Model file for the job. Use its own axes, mm. A direction names the side the tool comes from. Coordinates: 2 decimals unless noted, no trailing zeros. Loops run counter-clockwise (first coordinate to the right, second up) from the corner with the lowest first, then second, coordinate; pieces in that order, holes last. Notation, with made-up numbers: (-30.5, 76) -> (12.5, 76) arc R25 ccw to (12.5, 113) -> close; hole circle Ø10 at (48, 87). An arc over 180 degrees is marked (long way). Use one line per item in the form item = value.
```python
from build123d import *

# Parameters (mm, degrees)
ESBO_O1_W                = 44
ESBO_O1_H                = 65
RESSALTO_EXTRUS_O1_DEPTH = 19
ESBO_O2_W                = 40
ESBO_O2_H                = 15
CORTE_EXTRUS_O1_DEPTH    = 20
ESBO_O3_W                = 40
ESBO_O3_H                = 1.8
CORTE_EXTRUS_O2_DEPTH    = 43
ESBO_O4_W                = 33
ESBO_O4_H                = 7.6
CORTE_EXTRUS_O3_DEPTH    = 43
ESBO_O5_W                = 3.5
ESBO_O5_H                = 7.6
RESSALTO_EXTRUS_O2_DEPTH = 20
ESBO_O6_W                = 33
ESBO_O6_H                = 5.6
CORTE_EXTRUS_O4_DEPTH    = 43
ESBO_O7_W                = 3.5
ESBO_O7_H                = 2
ESBO_O7_W_2              = 40
CORTE_EXTRUS_O5_DEPTH    = 63
ESBO_O8_R                = 2.05
CORTE_EXTRUS_O6_DEPTH    = 3
ESBO_O9_W                = 3.5
ESBO_O9_H                = 7.601315145
CORTE_EXTRUS_O7_DEPTH    = 4
ESBO_O10_W               = 3.5
ESBO_O10_H               = 2
CORTE_EXTRUS_O9_DEPTH    = 16
ESBO_O12_W               = 8.25
ESBO_O12_H               = 4
ESBO_O12_W_2             = 4
ESBO_O12_H_2             = 7.625
RESSALTO_EXTRUS_O3_DEPTH = 8
CORTE_EXTRUS_O10_DEPTH   = 40
CORTE_EXTRUS_O11_DEPTH   = 24
RESSALTO_EXTRUS_O4_DEPTH = 1.8
ESBO_O18_W               = 3.925
ESBO_O18_H               = 5.6
RESSALTO_EXTRUS_O5_DEPTH = 2
CORTE_EXTRUS_O12_DEPTH   = 10
ESBO_O20_R               = 1.4
CORTE_EXTRUS_O13_DEPTH   = 16
ESBO_O21_W               = 3.925
ESBO_O21_H               = 7.6
RESSALTO_EXTRUS_O6_DEPTH = 2
CORTE_EXTRUS_O14_DEPTH   = 5
ESBO_O24_R               = 1.4
CORTE_EXTRUS_O15_DEPTH   = 16
ESBO_O26_W               = 20
ESBO_O26_H               = 2
CORTE_EXTRUS_O16_DEPTH   = 4
FILETE1_R                = 1


with BuildPart() as part:
    # Esboço1 → Ressalto-extrusão1 (new body)
    with BuildSketch(Plane(origin=(0, 0, 0), x_dir=(1, 0, 0), z_dir=(0, 1, 0))):
        Rectangle(ESBO_O1_W, ESBO_O1_H)
    extrude(amount=RESSALTO_EXTRUS_O1_DEPTH)

    # Esboço2 → Corte-extrusão1 (cut)
    with BuildSketch(Plane(origin=(0, 0, -32.5), x_dir=(-1, 0, 0), z_dir=(0, 0, -1))):
        with Locations((0, 9.5)):
            Rectangle(ESBO_O2_W, ESBO_O2_H)
    extrude(amount=-CORTE_EXTRUS_O1_DEPTH, mode=Mode.SUBTRACT)

    # Esboço3 → Corte-extrusão2 (cut)
    with BuildSketch(Plane(origin=(0, 0, -12.5), x_dir=(-1, 0, 0), z_dir=(0, 0, -1))):
        with Locations((0, 10.5)):
            Rectangle(ESBO_O3_W, ESBO_O3_H)
    extrude(amount=-CORTE_EXTRUS_O2_DEPTH, mode=Mode.SUBTRACT)

    # Esboço4 → Corte-extrusão3 (cut)
    with BuildSketch(Plane(origin=(0, 0, -12.5), x_dir=(-1, 0, 0), z_dir=(0, 0, -1))):
        with Locations((0, 5.8)):
            Rectangle(ESBO_O4_W, ESBO_O4_H)
    extrude(amount=-CORTE_EXTRUS_O3_DEPTH, mode=Mode.SUBTRACT)

    # Esboço5 → Ressalto-extrusão2 (add)
    with BuildSketch(Plane(origin=(0, 0, -12.5), x_dir=(-1, 0, 0), z_dir=(0, 0, -1))):
        with Locations((-18.25, 5.8)):
            Rectangle(ESBO_O5_W, ESBO_O5_H)
        with Locations((18.25, 5.8)):
            Rectangle(ESBO_O5_W, ESBO_O5_H)
    extrude(amount=RESSALTO_EXTRUS_O2_DEPTH)

    # Esboço6 → Corte-extrusão4 (cut)
    with BuildSketch(Plane(origin=(0, 0, -12.5), x_dir=(-1, 0, 0), z_dir=(0, 0, -1))):
        with Locations((0, 14.2)):
            Rectangle(ESBO_O6_W, ESBO_O6_H)
    extrude(amount=-CORTE_EXTRUS_O4_DEPTH, mode=Mode.SUBTRACT)

    # Esboço7 → Corte-extrusão5 (cut)
    with BuildSketch(Plane(origin=(0, 0, -32.5), x_dir=(-1, 0, 0), z_dir=(0, 0, -1))):
        with Locations((-18.25, 14.2)):
            Rectangle(ESBO_O7_W, ESBO_O7_H)
        with Locations((18.25, 14.2)):
            Rectangle(ESBO_O7_W, ESBO_O7_H)
        with Locations((0, 18)):
            Rectangle(ESBO_O7_W_2, ESBO_O7_H)
    extrude(amount=-CORTE_EXTRUS_O5_DEPTH, mode=Mode.SUBTRACT)

    # Esboço8 → Corte-extrusão6 (cut, through all)
    with BuildSketch(Plane(origin=(0, 2, 0), x_dir=(1, 0, 0), z_dir=(0, 1, 0))):
        with Locations((0, 16.25)):
            Circle(ESBO_O8_R)
        with Locations((0, -15.25)):
            Circle(ESBO_O8_R)
    extrude(amount=-CORTE_EXTRUS_O6_DEPTH, mode=Mode.SUBTRACT)

    # Esboço9 → Corte-extrusão7 (cut)
    with BuildSketch(Plane(origin=(0, 0, -32.5), x_dir=(-1, 0, 0), z_dir=(0, 0, -1))):
        with Locations((18.25, 5.799342428)):
            Rectangle(ESBO_O9_W, ESBO_O9_H)
        with Locations((-18.25, 5.799342428)):
            Rectangle(ESBO_O9_W, ESBO_O9_H)
    extrude(amount=-CORTE_EXTRUS_O7_DEPTH, mode=Mode.SUBTRACT)

    # Esboço10 → Corte-extrusão9 (cut)
    with BuildSketch(Plane(origin=(0, 0, -28.5), x_dir=(-1, 0, 0), z_dir=(0, 0, -1))):
        with Locations((-18.25, 8.6)):
            Rectangle(ESBO_O10_W, ESBO_O10_H)
    extrude(amount=-CORTE_EXTRUS_O9_DEPTH, mode=Mode.SUBTRACT)

    # Esboço12 → Ressalto-extrusão3 (add)
    with BuildSketch(Plane(origin=(0, 2, 0), x_dir=(1, 0, 0), z_dir=(0, 1, 0))):
        with Locations((12.375, 24.375)):
            Rectangle(ESBO_O12_W, ESBO_O12_H)
        with Locations((12.375, -7.625)):
            Rectangle(ESBO_O12_W, ESBO_O12_H)
        with Locations((8.25, -26.6875)):
            Rectangle(ESBO_O12_W_2, ESBO_O12_H_2)
        with Locations((-8.25, -26.6875)):
            Rectangle(ESBO_O12_W_2, ESBO_O12_H_2)
        with Locations((-12.375, -7.625)):
            Rectangle(ESBO_O12_W, ESBO_O12_H)
        with Locations((-12.375, 24.375)):
            Rectangle(ESBO_O12_W, ESBO_O12_H)
    extrude(amount=RESSALTO_EXTRUS_O3_DEPTH)

    # Esboço13 → Corte-extrusão10 (cut)
    with BuildSketch(Plane(origin=(0, 0, -26.375), x_dir=(-1, 0, 0), z_dir=(0, 0, -1))):
        Polygon((-8.25, 10), (-8.25, 2), (-16.5, 9.6), (-16.5, 10), align=None)
        Polygon((8.25, 2), (16.5, 9.6), (16.5, 10), (8.25, 10), align=None)
    extrude(amount=-CORTE_EXTRUS_O10_DEPTH, mode=Mode.SUBTRACT)

    # Esboço14 → Corte-extrusão11 (cut)
    with BuildSketch(Plane.ZY.offset(10.25)):
        Polygon((22.875, 2), (30.5, 9.625), (30.5, 10), (22.875, 10), align=None)
    extrude(amount=-CORTE_EXTRUS_O11_DEPTH, mode=Mode.SUBTRACT)

    # Esboço17 → Ressalto-extrusão4 (add)
    with BuildSketch(Plane(origin=(0, 0, -28.5), x_dir=(-1, 0, 0), z_dir=(0, 0, -1))):
        Polygon((-16.5, 2), (-16.5, 7.6), (-20, 7.6), (-20, 1.998684855), (-16.5, 1.998684855), align=None)
        Polygon((16.5, 9.6), (16.5, 2), (16.5, 1.998684855), (20, 1.998684855), (20, 9.6), align=None)
    extrude(amount=RESSALTO_EXTRUS_O4_DEPTH)

    # Esboço18 → Ressalto-extrusão5 (add)
    with BuildSketch(Plane.ZY.offset(-16.5)):
        with Locations((-28.3375, 4.8)):
            Rectangle(ESBO_O18_W, ESBO_O18_H)
    extrude(amount=RESSALTO_EXTRUS_O5_DEPTH)

    # Esboço19 → Corte-extrusão12 (cut)
    with BuildSketch(Plane(origin=(0, 0, -26.375), x_dir=(-1, 0, 0), z_dir=(0, 0, -1))):
        Polygon((-16.5, 9.6), (-16.5, 7.6), (-14.285160283, 7.559662806), align=None)
    extrude(amount=-CORTE_EXTRUS_O12_DEPTH, mode=Mode.SUBTRACT)

    # Esboço20 → Corte-extrusão13 (cut)
    with BuildSketch(Plane(origin=(0, 0, -30.3), x_dir=(-1, 0, 0), z_dir=(0, 0, -1))):
        with Locations((-17.25, 4.799342428)):
            Circle(ESBO_O20_R)
    extrude(amount=-CORTE_EXTRUS_O13_DEPTH, mode=Mode.SUBTRACT)

    # Esboço21 → Ressalto-extrusão6 (add)
    with BuildSketch(Plane(origin=(-16.5, 0, 0), x_dir=(0, 0, -1), z_dir=(1, 0, 0))):
        with Locations((28.3375, 5.8)):
            Rectangle(ESBO_O21_W, ESBO_O21_H)
    extrude(amount=RESSALTO_EXTRUS_O6_DEPTH)

    # Esboço23 → Corte-extrusão14 (cut)
    with BuildSketch(Plane(origin=(0, 0, -30.3), x_dir=(-1, 0, 0), z_dir=(0, 0, -1))):
        Polygon((13.624579494, 6.951127777), (17.102092839, 10.154655221), (13.624579494, 10.154655221), align=None)
    extrude(amount=-CORTE_EXTRUS_O14_DEPTH, mode=Mode.SUBTRACT)

    # Esboço24 → Corte-extrusão15 (cut)
    with BuildSketch(Plane(origin=(0, 0, -30.3), x_dir=(-1, 0, 0), z_dir=(0, 0, -1))):
        with Locations((17.25, 4.8)):
            Circle(ESBO_O24_R)
    extrude(amount=-CORTE_EXTRUS_O15_DEPTH, mode=Mode.SUBTRACT)

    # Esboço26 → Corte-extrusão16 (cut)
    with BuildSketch(Plane(origin=(0, 0, -32.5), x_dir=(-1, 0, 0), z_dir=(0, 0, -1))):
        with Locations((0, 1)):
            Rectangle(ESBO_O26_W, ESBO_O26_H)
    extrude(amount=-CORTE_EXTRUS_O16_DEPTH, mode=Mode.SUBTRACT)

    # Filete1
    filete1_edges = [part.edges().sort_by_distance(p)[0] for p in [
        (22, 9.5, 32.5),
        (-22, 9.5, 32.5),
    ]]
    fillet(filete1_edges, radius=FILETE1_R)


solid = part.part
```
Q1. Band-saw the part on D-D, the plane z = 4. Write the cut outline in (x, y).
Result:
outline = (-22, 0) -> (22, 0) -> (22, 19) -> (20, 19) -> (20, 17) -> (16.5, 17) -> (16.5, 15.2) -> (20, 15.2) -> (20, 13.2) -> (16.5, 13.2) -> (16.5, 11.4) -> (20, 11.4) -> (20, 9.6) -> (16.5, 9.6) -> (16.5, 2) -> (-16.5, 2) -> (-16.5, 9.6) -> (-20, 9.6) -> (-20, 11.4) -> (-16.5, 11.4) -> (-16.5, 13.2) -> (-20, 13.2) -> (-20, 15.2) -> (-16.5, 15.2) -> (-16.5, 17) -> (-20, 17) -> (-20, 19) -> (-22, 19) -> close
Q2. Wall check: line 1 along Z through (x, y) = (0, 0.8); line 2 along Z through (x, y) = (10.5, 3.5) (3 decimals); line 3 along X through (y, z) = (15.75, 8). Give the ranges that are in metal, low to high.
Result:
line_1 = -28.5 to -18.3, -14.2 to 13.2, 17.3 to 32.5
line_2 = -26.375 to -22.375, 5.625 to 9.625, 30.5 to 32.5
line_3 = -22 to -16.5, 16.5 to 22
Q3. Band-saw the part on A-A, the plane x = 0. Write the cut outline in (y, z), and give its area (3 significant figures).
Result:
outline = (0, -28.5) -> (2, -28.5) -> (2, -18.3) -> (0, -18.3) -> close; (0, -14.2) -> (2, -14.2) -> (2, 13.2) -> (0, 13.2) -> close; (0, 17.3) -> (2, 17.3) -> (2, 30.5) -> (19, 30.5) -> (19, 32.5) -> (0, 32.5) -> close
area = 140 mm2
Q4. Band-saw the part on C-C, the plane x = 17.25. Write the cut outline in (y, z), and give its area (3 significant figures).
Result:
outline = (0, -32.5) -> (2, -32.5) -> (2, -30.3) -> (3.4, -30.3) -> (3.4, -14.3) -> (6.2, -14.3) -> (6.2, -30.3) -> (7.6, -30.3) -> (7.6, -12.5) -> (9.6, -12.5) -> (9.6, 30.5) -> (11.4, 30.5) -> (11.4, -12.5) -> (13.2, -12.5) -> (13.2, 30.5) -> (15.2, 30.5) -> (15.2, -12.5) -> (17, -12.5) -> (17, 30.5) -> (19, 30.5) -> (19, 32.5) -> (0, 32.5) -> close
area = 700 mm2
Q5. Which spindle directions (+Z, -Z, +X, -X, +Y, -Y) get a long thin tool onto all of the face, cutting with end or side? Do faces 1 (the face through (-14.5, 5, -28)), 2 (the face through (-18, 9.6, 1)), 3 (the face through (14, 4, 5.625)), 4 (the face through (-0.444, 1.014, 17.251)), 5 (the face through (10, 1, -31)). Say none if no direction does.
Result:
face_1 = -Z, +Y
face_2 = -Z
face_3 = +Y
face_4 = +Y, -Y
face_5 = -Z, +Y, -Y
Q6. Pin check, flat tips, straight feed: pin 1 Ø4 at (x, y) = (-8, 5.5) entering from -Z (3 decimals); pin 2 Ø1.6 at (x, y) = (0.5, 0.5) entering from -Z; pin 3 Ø3 at (x, y) = (-15.5, 4.5) entering from -Z. Stop position of each tip, or through.
Result:
pin_1 = 24.375
pin_2 = -28.5
pin_3 = -30.3
